Input: part model. Units: mm. Frame: model coordinates. A direction names the side the tool comes from. Coordinates: 2 decimals unless noted, no trailing zeros. Order: outer loops, then holes, each group sorted by start corner. A loop starts at its lowest first (then second) coordinate and runs counter-clockwise, first axis right, second up. Notation, with made-up numbers: (-32.75, 30.5) - (3.25, 30.5) arc R26 ccw to (3.25, 69.5) - close; hole circle Ø4 at (79, 38.5). An arc over 180 degrees is marked (long way). Answer as CSV lines item,"result". Start each with the question number.
Item 1: First-contact query: pin 1 (4 mm diameter, centred on x = 0.5, z = -2, fed in from +Y); pin 2 (1.1 mm diameter, centred on y = 10.5, z = -12.5, fed in from -X); pin 3 (1.5 mm diameter, centred on x = 0, y = 14.224, fed in from -Z). Flat tips, straight axial feed; report the tip coordinate or a pass-through.
Item 2: Material intervals for line 1 along Y through (x, z) = (0, 2); line 2 along X through (y, z) = (21, -3); line 3 along Z through (x, y) = (2, 16.5) (3 decimals), sorted ascending.
Item 3: Section A-A (x = -10.5). Output: boundary loops of the cut face in (y, z) (3 decimals).
Item 4: Access query for faces 4 (the flat face through (-8, 38.1, 0)), 5 (the cylindrical face through (-1.64, 19.59, -5.21)), 6 (the flat face through (-5.08, 12, -13)). Directions: +Z, -Z, +X, -X, +Y, -Y. A direction counts if a zero-diameter tool reaches every point of the face in a straight line with its end or side. Return the directions, or none.
Item 5: Section C-C (z = 0). State how many separate pieces and enclosed holes the cut face has, and give its area (3 significant figures).
Item 6: Section B-B (y = 2). Output: boundary loops of the cut face in (x, z) (3 decimals), and give its area (3 significant figures).
Item 7: Draft query along Y for faces 1 (the flat face through (19.05, 19, 0)), 2 (the cylindrical face through (-0.888, 23.414, -10.911)), 3 (the cylindrical face through (-0.1, 27.1, -12.7)). Return one class per face: +Y half, -Y half, draft (parallel to the pull), parting line (faces both ways), or undercut.
from build123d import *

# Parameters (mm, degrees)
SKETCH1_W           = 38.1
SKETCH1_H           = 19.05
BOSS_EXTRUDE1_DEPTH = 12.7
SKETCH2_W           = 38.1
SKETCH2_H           = 19.05
SKETCH2_R           = 6.5405
BOSS_EXTRUDE2_DEPTH = 25.4
SKETCH2_3_R         = 5.461
BOSS_EXTRUDE3_DEPTH = 15.24
SKETCH3_R           = 0.635
SKETCH3_R_2         = 1.651
CUT_EXTRUDE1_DEPTH  = 47.6627796
BOSS_EXTRUDE4_START = 6.35
SKETCH4_R           = 0.635
SKETCH4_R_2         = 1.651
BOSS_EXTRUDE4_DEPTH = 6.35
FILLET3_R           = 1.27
FILLET4_R           = 1.27
CHAMFER1_SIZE       = 0.381
CHAMFER2_SIZE       = 0.508


with BuildPart() as part:
    # Sketch1 → Boss-Extrude1 (new body)
    with BuildSketch(Plane(origin=(0, 0, 0), x_dir=(1, 0, 0), z_dir=(0, 1, 0))):
        Rectangle(SKETCH1_W, SKETCH1_H)
    extrude(amount=BOSS_EXTRUDE1_DEPTH)

    # Sketch2 → Boss-Extrude2 (add)
    # profile 1 of 4: a face of its own
    with BuildSketch(Plane(origin=(0, 12.7, 0), x_dir=(1, 0, 0), z_dir=(0, 1, 0))):
        Rectangle(SKETCH2_W, SKETCH2_H)
        with Locations(Location((0, 0, 0), (0, 0, 270))):
            Circle(SKETCH2_R, mode=Mode.SUBTRACT)
    # profile 2 of 4: a face of its own
    with BuildSketch(Plane(origin=(0, 12.7, 0), x_dir=(1, 0, 0), z_dir=(0, 1, 0))):
        Rectangle(SKETCH2_W, SKETCH2_H)
        with Locations(Location((0, 0, 0), (0, 0, 270))):
            Circle(SKETCH2_R, mode=Mode.SUBTRACT)
    # profile 3 of 4: a face of its own
    with BuildSketch(Plane(origin=(0, 12.7, 0), x_dir=(1, 0, 0), z_dir=(0, 1, 0))):
        Rectangle(SKETCH2_W, SKETCH2_H)
        with Locations(Location((0, 0, 0), (0, 0, 270))):
            Circle(SKETCH2_R, mode=Mode.SUBTRACT)
    # profile 4 of 4: a face of its own
    with BuildSketch(Plane(origin=(0, 12.7, 0), x_dir=(1, 0, 0), z_dir=(0, 1, 0))):
        Rectangle(SKETCH2_W, SKETCH2_H)
        with Locations(Location((0, 0, 0), (0, 0, 270))):
            Circle(SKETCH2_R, mode=Mode.SUBTRACT)
    extrude(amount=BOSS_EXTRUDE2_DEPTH)

    # Sketch2<3> → Boss-Extrude3 (add)
    with BuildSketch(Plane(origin=(0, 12.7, 0), x_dir=(1, 0, 0), z_dir=(0, 1, 0))):
        with Locations(Location((0, 0, 0), (0, 0, 90))):
            Circle(SKETCH2_3_R)
    extrude(amount=BOSS_EXTRUDE3_DEPTH)

    # Sketch3 → Cut-Extrude1 (cut, through all)
    with BuildSketch(Plane(origin=(0, 0, -9.525), x_dir=(-1, 0, 0), z_dir=(0, 0, -1))):
        with Locations((0, 14.224)):
            Circle(SKETCH3_R)
        with Locations((0, 22.0218)):
            Circle(SKETCH3_R_2)
    extrude(amount=-CUT_EXTRUDE1_DEPTH, mode=Mode.SUBTRACT)

    # Sketch4 → Boss-Extrude4 (add)
    with BuildSketch(Plane(origin=(0, 0, -9.525), x_dir=(-1, 0, 0), z_dir=(0, 0, -1)).offset(BOSS_EXTRUDE4_START)):
        with BuildLine():
            Line((5.08, 0), (5.08, 22.0218))
            ThreePointArc((5.08, 22.0218), (0, 27.1018), (-5.08, 22.0218))
            Line((-5.08, 22.0218), (-5.08, 0))
            Line((-5.08, 0), (5.08, 0))
        make_face()
        with Locations((0, 14.224)):
            Circle(SKETCH4_R, mode=Mode.SUBTRACT)
        with Locations((0, 22.0218)):
            Circle(SKETCH4_R_2, mode=Mode.SUBTRACT)
    extrude(amount=-BOSS_EXTRUDE4_DEPTH)

    # Fillet3
    fillet3_edges = [part.edges().sort_by_distance(p)[0] for p in [
        (0, 38.1, -6.5405),
        (0, 38.1, 9.525),
        (19.05, 38.1, 0),
        (0, 38.1, -9.525),
        (-19.05, 38.1, 0),
        (0, 0, 9.525),
        (-19.05, 0, 0),
        (-12.065, 0, -9.525),
        (12.065, 0, -9.525),
        (-5.08, 11.0109, -15.875),
        (-5.08, 0, -12.7),
        (0, 27.1018, -9.525),
        (5.08, 11.0109, -9.525),
        (5.08, 0, -12.7),
        (0, 27.1018, -15.875),
        (5.08, 11.0109, -15.875),
        (19.05, 0, 0),
        (0, 0, -15.875),
        (-5.08, 11.0109, -9.525),
        (19.05, 19.05, 9.525),
        (-19.05, 19.05, 9.525),
        (-19.05, 19.05, -9.525),
        (19.05, 19.05, -9.525),
    ]]
    fillet(fillet3_edges, radius=FILLET3_R)

    # Fillet4
    fillet4_edges = [part.edges().sort_by_distance(p)[0] for p in [
        (0, 27.94, 5.461),
    ]]
    fillet(fillet4_edges, radius=FILLET4_R)

    # Chamfer1
    chamfer1_edges = [part.edges().sort_by_distance(p)[0] for p in [
        (0.635, 14.224, -15.875),
    ]]
    chamfer(chamfer1_edges, length=CHAMFER1_SIZE)

    # Chamfer2
    chamfer2_edges = [part.edges().sort_by_distance(p)[0] for p in [
        (1.651, 22.0218, -15.875),
    ]]
    chamfer(chamfer2_edges, length=CHAMFER2_SIZE)


solid = part.part
Determined:
1,pin 1,"stops at y = 27.94"
1,pin 2,"stops at x = -5.08"
1,pin 3,"stops at z = -15.61"
2,line 1,"y = 0 to 13.59, 14.86 to 20.37, 23.67 to 27.94"
2,line 2,"x = -19.05 to -5.81, -4.56 to -1.3, 1.3 to 4.56, 5.81 to 19.05"
2,line 3,"z = -15.875 to -6.227, -5.082 to 5.082, 6.227 to 9.525"
3,outline,"(0, -8.255) arc R1.27 ccw to (1.27, -9.525) - (36.83, -9.525) arc R1.27 ccw to (38.1, -8.255) - (38.1, 8.255) arc R1.27 ccw to (36.83, 9.525) - (1.27, 9.525) arc R1.27 ccw to (0, 8.255) - close"
4,face 4,"+Z, -Z, +X, -X, +Y"
4,face 5,"+Y"
4,face 6,"-Z, -X, +Y, -Y"
5,separate pieces,"1"
5,enclosed holes,"2"
5,area,"1,270 mm^2"
6,outline,"(-19.05, -8.255) arc R1.27 ccw to (-17.78, -9.525) - (-6.35, -9.525) arc R1.27 cw to (-5.08, -10.795) - (-5.08, -14.605) arc R1.27 ccw to (-3.81, -15.875) - (3.81, -15.875) arc R1.27 ccw to (5.08, -14.605) - (5.08, -10.795) arc R1.27 cw to (6.35, -9.525) - (17.78, -9.525) arc R1.27 ccw to (19.05, -8.255) - (19.05, 8.255) arc R1.27 ccw to (17.78, 9.525) - (-17.78, 9.525) arc R1.27 ccw to (-19.05, 8.255) - close"
6,area,"789 mm^2"
7,face 1,"draft"
7,face 2,"undercut"
7,face 3,"+Y half"
